from build123d import *

# Parameters (mm, degrees)
CUT_EXTRUDE1_OUTLINE_R   = 2.0701
CUT_EXTRUDE1_DEPTH       = 3.0988
CUT_EXTRUDE1_START       = 2.286
CUT_EXTRUDE1_2_OUTLINE_W = 2.286
CUT_EXTRUDE1_2_OUTLINE_H = 152.4
CUT_EXTRUDE1_2_DEPTH     = 48.514
CUT_EXTRUDE1_START_2     = 3.0988
CUT_EXTRUDE1_3_OUTLINE_W = 0.8128
CUT_EXTRUDE1_3_OUTLINE_H = 152.4
CUT_EXTRUDE1_3_DEPTH     = 47.7012
CUT_EXTRUDE1_4_OUTLINE_R = 2.0701
CUT_EXTRUDE1_4_DEPTH     = 2.286
CUT_EXTRUDE1_START_3     = -749.3
CUT_EXTRUDE1_5_DEPTH     = 152.4
CUT_EXTRUDE1_START_4     = 564.229492087
CUT_EXTRUDE1_6_OUTLINE_W = 5
CUT_EXTRUDE1_6_OUTLINE_H = 6
CUT_EXTRUDE1_6_DEPTH     = 2.770507913
CHAMFER1_SIZE            = 2.159
BOSS_EXTRUDE1_START      = -2.286
BOSS_EXTRUDE1_DEPTH      = 2.286
BOSS_EXTRUDE2_START      = -2.286
BOSS_EXTRUDE2_DEPTH      = 2.286
SKETCH4_W                = 50.8
SKETCH4_H                = 50.8
CUT_EXTRUDE2_DEPTH       = 12.7
SKETCH5_W                = 50.8
SKETCH5_H                = 50.8
CUT_EXTRUDE3_DEPTH       = 12.7
BOSS_EXTRUDE3_START      = -2.286
BOSS_EXTRUDE3_DEPTH      = 2.286
BOSS_EXTRUDE4_START      = -2.286
BOSS_EXTRUDE4_DEPTH      = 2.286
CHAMFER2_SIZE            = 2.159


with BuildPart() as part:
    # Cut-Extrude1: read off the stored shape, not the designer's step
    # Cut-Extrude1 outline → Cut-Extrude1 (new body)
    with BuildSketch(Plane(origin=(0, 0, 0), x_dir=(1, 0, 0), z_dir=(0, 1, 0))):
        with BuildLine():
            ThreePointArc((23.3299, 596.9), (23.936218252, 598.363781748), (25.4, 598.9701))
            ThreePointArc((25.4, 598.9701), (26.863781748, 598.363781748), (27.4701, 596.9))
            Line((27.4701, 596.9), (50.8, 596.9))
            Line((50.8, 596.9), (50.8, 747.141))
            Line((50.8, 747.141), (48.641, 749.3))
            Line((48.641, 749.3), (0, 749.3))
            Line((0, 749.3), (0, 596.9))
            Line((0, 596.9), (23.3299, 596.9))
        make_face()
        with Locations((12.7, 609.6)):
            Circle(CUT_EXTRUDE1_OUTLINE_R, mode=Mode.SUBTRACT)
        with Locations((25.4, 622.3)):
            Circle(CUT_EXTRUDE1_OUTLINE_R, mode=Mode.SUBTRACT)
        with Locations((12.7, 635)):
            Circle(CUT_EXTRUDE1_OUTLINE_R, mode=Mode.SUBTRACT)
        with Locations((12.7, 660.4)):
            Circle(CUT_EXTRUDE1_OUTLINE_R, mode=Mode.SUBTRACT)
        with Locations((25.4, 647.7)):
            Circle(CUT_EXTRUDE1_OUTLINE_R, mode=Mode.SUBTRACT)
        with Locations((38.1, 609.6)):
            Circle(CUT_EXTRUDE1_OUTLINE_R, mode=Mode.SUBTRACT)
        with Locations((38.1, 635)):
            Circle(CUT_EXTRUDE1_OUTLINE_R, mode=Mode.SUBTRACT)
        with Locations((38.1, 660.4)):
            Circle(CUT_EXTRUDE1_OUTLINE_R, mode=Mode.SUBTRACT)
        with Locations((12.7, 685.8)):
            Circle(CUT_EXTRUDE1_OUTLINE_R, mode=Mode.SUBTRACT)
        with Locations((25.4, 673.1)):
            Circle(CUT_EXTRUDE1_OUTLINE_R, mode=Mode.SUBTRACT)
        with Locations((25.4, 698.5)):
            Circle(CUT_EXTRUDE1_OUTLINE_R, mode=Mode.SUBTRACT)
        with Locations((12.7, 711.2)):
            Circle(CUT_EXTRUDE1_OUTLINE_R, mode=Mode.SUBTRACT)
        with Locations((12.7, 736.6)):
            Circle(CUT_EXTRUDE1_OUTLINE_R, mode=Mode.SUBTRACT)
        with Locations((25.4, 723.9)):
            Circle(CUT_EXTRUDE1_OUTLINE_R, mode=Mode.SUBTRACT)
        with Locations((38.1, 685.8)):
            Circle(CUT_EXTRUDE1_OUTLINE_R, mode=Mode.SUBTRACT)
        with Locations((38.1, 711.2)):
            Circle(CUT_EXTRUDE1_OUTLINE_R, mode=Mode.SUBTRACT)
        with Locations((38.1, 736.6)):
            Circle(CUT_EXTRUDE1_OUTLINE_R, mode=Mode.SUBTRACT)
    extrude(amount=CUT_EXTRUDE1_DEPTH)

    # Cut-Extrude1 2 outline → Cut-Extrude1 2 (add)
    with BuildSketch(Plane(origin=(0, 0, 0), x_dir=(1, 0, 0), z_dir=(0, 1, 0)).offset(CUT_EXTRUDE1_START)):
        with Locations((1.143, 673.1)):
            Rectangle(CUT_EXTRUDE1_2_OUTLINE_W, CUT_EXTRUDE1_2_OUTLINE_H)
    extrude(amount=CUT_EXTRUDE1_2_DEPTH)

    # Cut-Extrude1 3 outline → Cut-Extrude1 3 (cut)
    with BuildSketch(Plane.YZ.offset(CUT_EXTRUDE1_START_2)):
        with Locations((2.6924, -673.1)):
            Rectangle(CUT_EXTRUDE1_3_OUTLINE_W, CUT_EXTRUDE1_3_OUTLINE_H)
    extrude(amount=CUT_EXTRUDE1_3_DEPTH, mode=Mode.SUBTRACT)

    # Cut-Extrude1 4 outline → Cut-Extrude1 4 (cut)
    with BuildSketch(Plane.YZ):
        with BuildLine():
            ThreePointArc((23.3299, -596.9), (23.936218252, -598.363781748), (25.4, -598.9701))
            ThreePointArc((25.4, -598.9701), (26.863781748, -598.363781748), (27.4701, -596.9))
            Line((27.4701, -596.9), (23.3299, -596.9))
        make_face()
        with Locations((25.4, -723.9)):
            Circle(CUT_EXTRUDE1_4_OUTLINE_R)
        with Locations((25.4, -698.5)):
            Circle(CUT_EXTRUDE1_4_OUTLINE_R)
        with Locations((25.4, -673.1)):
            Circle(CUT_EXTRUDE1_4_OUTLINE_R)
        with Locations((25.4, -647.7)):
            Circle(CUT_EXTRUDE1_4_OUTLINE_R)
        with Locations((25.4, -622.3)):
            Circle(CUT_EXTRUDE1_4_OUTLINE_R)
        with Locations((12.7, -736.6)):
            Circle(CUT_EXTRUDE1_4_OUTLINE_R)
        with Locations((12.7, -711.2)):
            Circle(CUT_EXTRUDE1_4_OUTLINE_R)
        with Locations((12.7, -685.8)):
            Circle(CUT_EXTRUDE1_4_OUTLINE_R)
        with Locations((12.7, -660.4)):
            Circle(CUT_EXTRUDE1_4_OUTLINE_R)
        with Locations((12.7, -635)):
            Circle(CUT_EXTRUDE1_4_OUTLINE_R)
        with Locations((12.7, -609.6)):
            Circle(CUT_EXTRUDE1_4_OUTLINE_R)
        with Locations((38.1, -736.6)):
            Circle(CUT_EXTRUDE1_4_OUTLINE_R)
        with Locations((38.1, -711.2)):
            Circle(CUT_EXTRUDE1_4_OUTLINE_R)
        with Locations((38.1, -685.8)):
            Circle(CUT_EXTRUDE1_4_OUTLINE_R)
        with Locations((38.1, -660.4)):
            Circle(CUT_EXTRUDE1_4_OUTLINE_R)
        with Locations((38.1, -635)):
            Circle(CUT_EXTRUDE1_4_OUTLINE_R)
        with Locations((38.1, -609.6)):
            Circle(CUT_EXTRUDE1_4_OUTLINE_R)
    extrude(amount=CUT_EXTRUDE1_4_DEPTH, mode=Mode.SUBTRACT)

    # Cut-Extrude1 5 outline → Cut-Extrude1 5 (cut)
    with BuildSketch(Plane.XY.offset(CUT_EXTRUDE1_START_3)):
        with BuildLine():
            ThreePointArc((3.0988, 0), (0.907617506, 0.907617506), (0, 3.0988))
            Line((0, 3.0988), (2.4e-08, 50))
            Line((2.4e-08, 50), (-1, 50))
            Line((-1, 50), (-1, -1))
            Line((-1, -1), (5, -1))
            Line((5, -1), (5, 1e-09))
            Line((5, 1e-09), (3.0988, 0))
        make_face()
        with BuildLine():
            Line((3.0988, 3.0988), (2.286, 3.0988))
            ThreePointArc((2.286, 3.0988), (2.524063608, 2.524063608), (3.0988, 2.286))
            Line((3.0988, 2.286), (3.0988, 3.0988))
        make_face()
    extrude(amount=CUT_EXTRUDE1_5_DEPTH, mode=Mode.SUBTRACT)

    # Cut-Extrude1 6 outline → Cut-Extrude1 6 (cut)
    with BuildSketch(Plane(origin=(0, 0, 0), x_dir=(1, 0, 0), z_dir=(0, 0.7071067811865511, -0.7071067811865441)).offset(CUT_EXTRUDE1_START_4)):
        with Locations((1.5, 494)):
            Rectangle(CUT_EXTRUDE1_6_OUTLINE_W, CUT_EXTRUDE1_6_OUTLINE_H)
    extrude(amount=CUT_EXTRUDE1_6_DEPTH, mode=Mode.SUBTRACT)

    # Chamfer1
    chamfer1_edges = [part.edges().sort_by_distance(p)[0] for p in [
        (1.143, 50.8, -596.9),
        (50.8, 1.143, -596.9),
    ]]
    chamfer(chamfer1_edges, length=CHAMFER1_SIZE)

    # Sketch2 → Boss-Extrude1 (add)
    with BuildSketch(Plane(origin=(2.286, 0, 0), x_dir=(0, 0, -1), z_dir=(1, 0, 0)).offset(BOSS_EXTRUDE1_START)):
        with BuildLine():
            Line((596.9, 27.4701), (596.9, 23.3299))
            ThreePointArc((596.9, 23.3299), (598.9701, 25.4), (596.9, 27.4701))
        make_face()
    extrude(amount=BOSS_EXTRUDE1_DEPTH)

    # Sketch3 → Boss-Extrude2 (add)
    with BuildSketch(Plane(origin=(0, 2.286, 0), x_dir=(1, 0, 0), z_dir=(0, 1, 0)).offset(BOSS_EXTRUDE2_START)):
        with BuildLine():
            Line((27.4701, 596.9), (23.3299, 596.9))
            ThreePointArc((23.3299, 596.9), (25.4, 598.9701), (27.4701, 596.9))
        make_face()
    extrude(amount=BOSS_EXTRUDE2_DEPTH)

    # Sketch4 → Cut-Extrude2 (cut)
    with BuildSketch(Plane.XY.offset(-596.9)):
        with Locations((25.4, 25.4)):
            Rectangle(SKETCH4_W, SKETCH4_H)
    extrude(amount=-CUT_EXTRUDE2_DEPTH, mode=Mode.SUBTRACT)

    # Sketch5 → Cut-Extrude3 (cut)
    with BuildSketch(Plane(origin=(0, 0, -749.3), x_dir=(-1, 0, 0), z_dir=(0, 0, -1))):
        with Locations((-25.4, 25.4)):
            Rectangle(SKETCH5_W, SKETCH5_H)
    extrude(amount=-CUT_EXTRUDE3_DEPTH, mode=Mode.SUBTRACT)

    # Sketch6 → Boss-Extrude3 (add)
    with BuildSketch(Plane(origin=(0, 2.286, 0), x_dir=(1, 0, 0), z_dir=(0, 1, 0)).offset(BOSS_EXTRUDE3_START)):
        with BuildLine():
            Line((40.1701, 609.6), (36.0299, 609.6))
            ThreePointArc((36.0299, 609.6), (36.636218252, 611.063781748), (38.1, 611.6701))
            ThreePointArc((38.1, 611.6701), (39.563781748, 611.063781748), (40.1701, 609.6))
        make_face()
        with BuildLine():
            Line((14.7701, 609.6), (10.6299, 609.6))
            ThreePointArc((10.6299, 609.6), (11.236218252, 611.063781748), (12.7, 611.6701))
            ThreePointArc((12.7, 611.6701), (14.163781748, 611.063781748), (14.7701, 609.6))
        make_face()
        with BuildLine():
            Line((40.1701, 736.6), (36.0299, 736.6))
            ThreePointArc((36.0299, 736.6), (36.636218252, 735.136218252), (38.1, 734.5299))
            ThreePointArc((38.1, 734.5299), (39.563781748, 735.136218252), (40.1701, 736.6))
        make_face()
        with BuildLine():
            Line((14.7701, 736.6), (10.6299, 736.6))
            ThreePointArc((10.6299, 736.6), (11.236218252, 735.136218252), (12.7, 734.5299))
            ThreePointArc((12.7, 734.5299), (14.163781748, 735.136218252), (14.7701, 736.6))
        make_face()
    extrude(amount=BOSS_EXTRUDE3_DEPTH)

    # Sketch7 → Boss-Extrude4 (add)
    with BuildSketch(Plane(origin=(2.286, 0, 0), x_dir=(0, 0, -1), z_dir=(1, 0, 0)).offset(BOSS_EXTRUDE4_START)):
        with BuildLine():
            Line((736.6, 10.6299), (736.6, 14.7701))
            ThreePointArc((736.6, 14.7701), (735.136218252, 14.163781748), (734.5299, 12.7))
            ThreePointArc((734.5299, 12.7), (735.136218252, 11.236218252), (736.6, 10.6299))
        make_face()
        with BuildLine():
            Line((736.6, 36.0299), (736.6, 40.1701))
            ThreePointArc((736.6, 40.1701), (735.136218252, 39.563781748), (734.5299, 38.1))
            ThreePointArc((734.5299, 38.1), (735.136218252, 36.636218252), (736.6, 36.0299))
        make_face()
        with BuildLine():
            Line((609.6, 10.6299), (609.6, 14.7701))
            ThreePointArc((609.6, 14.7701), (611.063781748, 14.163781748), (611.6701, 12.7))
            ThreePointArc((611.6701, 12.7), (611.063781748, 11.236218252), (609.6, 10.6299))
        make_face()
        with BuildLine():
            Line((609.6, 36.0299), (609.6, 40.1701))
            ThreePointArc((609.6, 40.1701), (611.063781748, 39.563781748), (611.6701, 38.1))
            ThreePointArc((611.6701, 38.1), (611.063781748, 36.636218252), (609.6, 36.0299))
        make_face()
    extrude(amount=BOSS_EXTRUDE4_DEPTH)

    # Chamfer2
    chamfer2_edges = [part.edges().sort_by_distance(p)[0] for p in [
        (50.8, 1.143, -609.6),
        (1.143, 50.8, -609.6),
        (1.143, 50.8, -736.6),
        (50.8, 1.143, -736.6),
    ]]
    chamfer(chamfer2_edges, length=CHAMFER2_SIZE)


solid = part.part
CAD build for the part. Positions are in the model's coordinates, mm. Coordinates: 2 decimals unless noted, no trailing zeros. Loops run counter-clockwise (first coordinate to the right, second up) from the corner with the lowest first, then second, coordinate; pieces in that order, holes last. Notation, with made-up numbers: (32.5, 0.5) - (50.5, 0.5) arc R31 ccw to (50.5, 25.5) - close; hole circle Ø10 at (87.25, -5). An arc over 180 degrees is marked (long way). Write item = value, one per line. Start each with the question number.
Q1. Cut at A-A, the plane z = -698.5. List the corners of the cut face in (x, y), then the cut area to 3 significant figures.
Q2. Pull direction Y, two halves, no side cores. Call faces 1 (the flat face through (33, 2.286, -674)), 2 (the flat face through (0, 33, -672)), 3 (the cylindrical face through (1.13, 37.65, -687.82)): pulls with the +Y half, pulls with the -Y half, needs draft (parallel to the pull), parting line crosses it, or undercut.
Q3. Cut at B-B, the plane x = 12.7. List the corners of the cut face in (y, z), then the cut area to 3 significant figures.
Q4. Flat gauge pins, fed straight in: pin 1 Ø3 at (y, z) = (27.5, -648) entering from -X; pin 2 Ø3 at (x, z) = (31.5, -722.5) entering from +Y; pin 3 Ø6 at (y, z) = (21.5, -706.5) entering from +X. Where does each tip first touch, or does it go through?
Q5. Cut at C-C, the plane y = 25.4. List the corners of the cut face in (x, z).
Q6. Cut at D-D, the plane z = -685.8. List the corners of the cut face in (x, y), then the cut area to 3 significant figures.
Q7. Drill centre lines: L1, parallel to Z at x = 12.7, y = 1.8; L2, parallel to X at y = 19.5, z = -696. Where is each one in solid material? Low to high.
Computed:
q1.outline = (0, 3.1) arc R3.1 ccw to (3.1, 0) - (23.33, 0) - (23.33, 2.29) - (3.1, 2.29) arc R0.81 cw to (2.29, 3.1) - (2.29, 23.33) - (0, 23.33) - close; (0, 27.47) - (2.29, 27.47) - (2.29, 50.8) - (0, 50.8) - close; (27.47, 0) - (50.8, 0) - (50.8, 2.29) - (27.47, 2.29) - close
q1.area = 206 mm²
q2.face_1 = pulls with the +Y half
q2.face_2 = needs draft
q2.face_3 = undercut
q3.outline = (0, -736.6) - (2.29, -736.6) - (2.29, -713.27) - (0, -713.27) - close; (0, -709.13) - (2.29, -709.13) - (2.29, -687.87) - (0, -687.87) - close; (0, -683.73) - (2.29, -683.73) - (2.29, -662.47) - (0, -662.47) - close; (0, -658.33) - (2.29, -658.33) - (2.29, -637.07) - (0, -637.07) - close; (0, -632.93) - (2.29, -632.93) - (2.29, -609.6) - (0, -609.6) - close
q3.area = 252 mm²
q4.pin_1 = 0
q4.pin_2 = 2.29
q4.pin_3 = 2.29
q5.outline = (0, -736.6) - (2.29, -736.6) - (2.29, -725.97) - (0, -725.97) - close; (0, -721.83) - (2.29, -721.83) - (2.29, -700.57) - (0, -700.57) - close; (0, -696.43) - (2.29, -696.43) - (2.29, -675.17) - (0, -675.17) - close; (0, -671.03) - (2.29, -671.03) - (2.29, -649.77) - (0, -649.77) - close; (0, -645.63) - (2.29, -645.63) - (2.29, -624.37) - (0, -624.37) - close; (0, -620.23) - (2.29, -620.23) - (2.29, -609.6) - (0, -609.6) - close
q6.outline = (0, 3.1) arc R3.1 ccw to (3.1, 0) - (10.63, 0) - (10.63, 2.29) - (3.1, 2.29) arc R0.81 cw to (2.29, 3.1) - (2.29, 10.63) - (0, 10.63) - close; (0, 14.77) - (2.29, 14.77) - (2.29, 36.03) - (0, 36.03) - close; (0, 40.17) - (2.29, 40.17) - (2.29, 50.8) - (0, 50.8) - close; (14.77, 0) - (36.03, 0) - (36.03, 2.29) - (14.77, 2.29) - close; (40.17, 0) - (50.8, 0) - (50.8, 2.29) - (40.17, 2.29) - close
q6.area = 187 mm²
q7.L1 = -736.6 to -713.27, -709.13 to -687.87, -683.73 to -662.47, -658.33 to -637.07, -632.93 to -609.6
q7.L2 = 0 to 2.29
